Design review of the part built by this model. Coordinates are the model's own, in mm. A direction names the side the tool comes from. Coordinates: 2 decimals unless noted, no trailing zeros. Loops run counter-clockwise (first coordinate to the right, second up) from the corner with the lowest first, then second, coordinate; pieces in that order, holes last. Notation, with made-up numbers: M -16.75,-9.75 L 27.25,-9.75 A19 cw 27.25,19.25 Z; hole C 52,-40 d10. An arc over 180 degrees is marked long. One line per item, written item: value.
```python
from build123d import *

# Parameters (mm, degrees)
F1_DEPTH = 144
F3_DEPTH = 1.001


# Not quite as in the source:
# - a feature names something its author has since deleted; it is built from what else it names


with BuildPart() as f1:
    # F0 (on Front) → F1 (new body)
    with BuildSketch(Plane.XZ):
        Polygon((-17.5, 6), (-17.5, 5), (-13.5, 5), (-13.5, -1), (13.5, -1), (13.5, 5), (17.5, 5), (17.5, 6), (12.5, 6), (12.5, 0), (-12.5, 0), (-12.5, 6), align=None)
    extrude(amount=F1_DEPTH)

    # F2 (on face) → F3 (cut, through all)
    with BuildSketch(Plane.XY):
        with BuildLine():
            ThreePointArc((-2.25, -28.25), (0, -30.5), (2.25, -28.25))
            Line((2.25, -28.25), (2.25, -7.75))
            ThreePointArc((2.25, -7.75), (0, -5.5), (-2.25, -7.75))
            Line((-2.25, -7.75), (-2.25, -28.25))
        make_face()
        with BuildLine():
            Line((-2.25, -43.75), (-2.25, -64.25))
            ThreePointArc((-2.25, -64.25), (0, -66.5), (2.25, -64.25))
            Line((2.25, -64.25), (2.25, -43.75))
            ThreePointArc((2.25, -43.75), (0, -41.5), (-2.25, -43.75))
        make_face()
        with BuildLine():
            Line((-2.25, -79.75), (-2.25, -100.25))
            ThreePointArc((-2.25, -100.25), (0, -102.5), (2.25, -100.25))
            Line((2.25, -100.25), (2.25, -79.75))
            ThreePointArc((2.25, -79.75), (0, -77.5), (-2.25, -79.75))
        make_face()
        with BuildLine():
            Line((-2.25, -115.75), (-2.25, -136.25))
            ThreePointArc((-2.25, -136.25), (0, -138.5), (2.25, -136.25))
            Line((2.25, -136.25), (2.25, -115.75))
            ThreePointArc((2.25, -115.75), (0, -113.5), (-2.25, -115.75))
        make_face()
    extrude(amount=-F3_DEPTH, mode=Mode.SUBTRACT)


solid = f1.part
```
(1) We need section A-A on y = -121.5. State the section outline as (x, z) points, then the cut area to 3 significant figures.
Reply:
outline: M -17.5,5 L -13.5,5 L -13.5,-1 L -2.25,-1 L -2.25,0 L -12.5,0 L -12.5,6 L -17.5,6 Z; M 2.25,-1 L 13.5,-1 L 13.5,5 L 17.5,5 L 17.5,6 L 12.5,6 L 12.5,0 L 2.25,0 Z
area: 42.5 mm2
(2) Insertion check: pin 1 (1.1 mm diameter, centred on y = -122.5, z = -0.5, fed in from +X); pin 2 (7.5 mm diameter, centred on x = -1, y = -95.5, fed in from +Z); pin 3 (3 mm diameter, centred on y = -107.5, z = 1.5, fed in from -X). Each pin has a flat end and moves straight along its axis. Give the tip position at first contact, or say it passes through.
Reply:
pin 1: stops at x = 13.5
pin 2: stops at z = 0
pin 3: stops at x = -13.5
(3) To check wall thickness, follow line 1 along X through (y, z) = (-66, 5.75); line 2 along X through (y, z) = (-85, 0.5); line 3 along Z through (x, y) = (-6, -91). State the ranges of each line that lie inside material, in increasing order. Write a range as [from, to].
Reply:
line 1: x = [-17.5, -12.5], [12.5, 17.5]
line 2: x = [-13.5, -12.5], [12.5, 13.5]
line 3: z = [-1, 0]
(4) We need section B-B on z = 2.75. State the section outline as (x, y) points.
Reply:
outline: M -13.5,-144 L -12.5,-144 L -12.5,0 L -13.5,0 Z; M 12.5,-144 L 13.5,-144 L 13.5,0 L 12.5,0 Z
(5) Tool access review of faces 5 (the flat face through (-0.1, 0, -0.3)), 6 (the flat face through (-12.5, -71, 3)), 7 (the cylindrical face through (0, -138.5, -0.5)), 8 (the flat face through (15, -71, 5)): name each direction out of +Z, -Z, +X, -X, +Y, -Y from which nothing blocks a thin tool from reaching the whole face with its end or side.
Reply:
face 5: +Z, -Z, +X, -X, +Y
face 6: +Z, +Y, -Y
face 7: +Z, -Z
face 8: -Z, +X, +Y, -Y
(6) We need section C-C on x = 4.5. State the section outline as (y, z) points.
Reply:
outline: M -144,-1 L 0,-1 L 0,0 L -144,0 Z
(7) Mouldability with a two-part tool opening along X and no side actions: class faces 1 (the cylindrical face through (0, -66.5, -0.5)), 2 (the flat face through (-13.5, -71, 2)), 3 (the flat face through (13.5, -71, 2)), 4 (the flat face through (15, -71, 6)) as released by +X, released by -X, zero draft, split by the parting line, or undercut.
Reply:
face 1: undercut
face 2: released by -X
face 3: released by +X
face 4: zero draft
